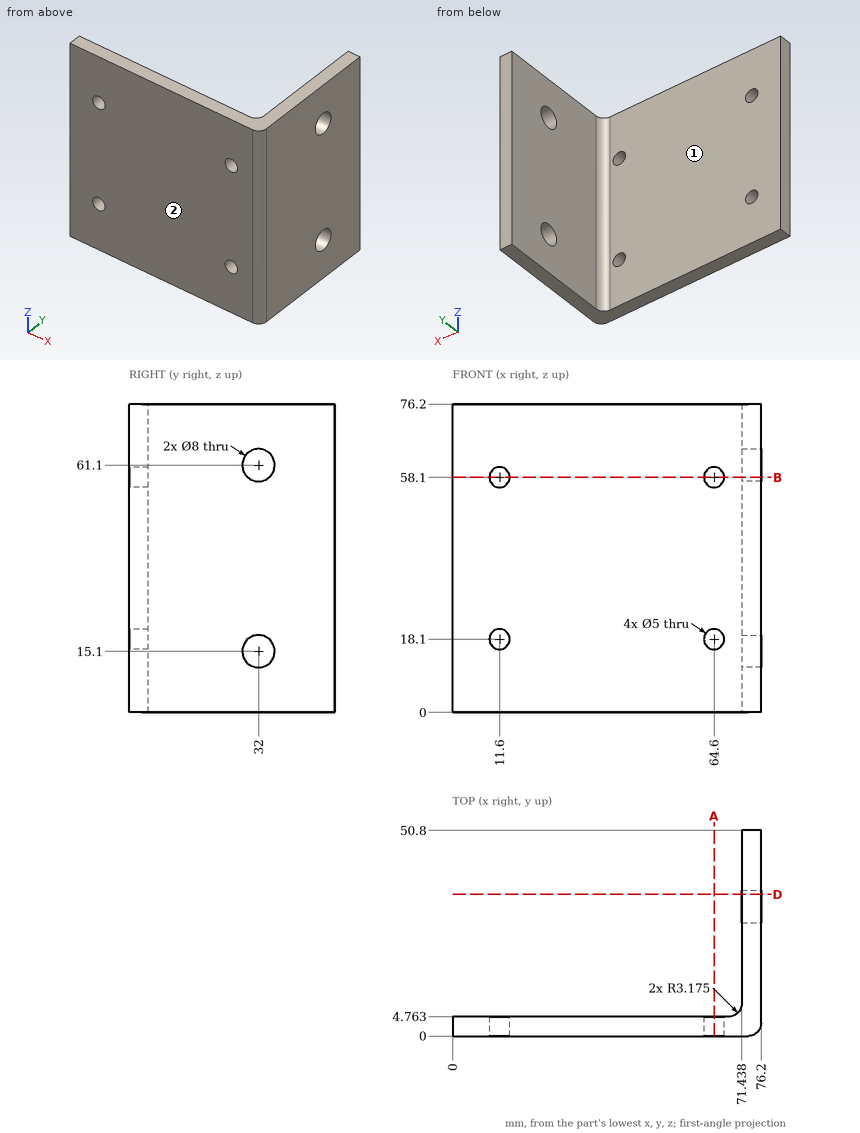
Can you work these out from the drawing? Everything is in mm from the part's minimum corner. A direction names the side the tool comes from. Coordinates: 2 decimals unless noted, no trailing zeros. Loops run counter-clockwise (first coordinate to the right, second up) from the corner with the lowest first, then second, coordinate; pieces in that order, holes last.
1. Imagine slicing it at A-A, the plane x = 64.6. Please give me the cut outline in (y, z).
2. Imagine slicing it at B-B, the plane z = 58.1. Count the separate pieces of the cut face and the enclosed holes in it.
3. Imagine slicing it at D-D, the plane y = 35. Please give me the cut outline in (x, z) (1 decimal).
4. I need wall thicknesses on L1, parallel to Z at x = 64.6, y = 1.85; L2, parallel to X at y = 3, z = 58 (1 decimal); L3, parallel to Z at x = 64, y = 2. Which ranges of each line are inside material? Lowest first, please.
5. For the marked faces 1 and 2, which set-ups out of +Z, -Z, +X, -X, +Y, -Y let a thin tool reach every point of the face, with its end or its side?
6. For P1, Ø1.5, axis at x = 61.5, z = 39, coming from the +Y side; P2, Ø6.5, axis at y = 32, z = 61.1, coming from the +X side; P3, Ø6, axis at x = 64.6, z = 18.1, coming from the -Y side; P4, Ø21.5, axis at y = 20, z = 32.5, coming from the -X side, each with a flat end and sliding along its axis, tell me the tip position at first contact or that it passes through.
Taken from the geometry:
1. outline: (0, 0) - (4.76, 0) - (4.76, 15.6) - (0, 15.6) - close; (0, 20.6) - (4.76, 20.6) - (4.76, 55.6) - (0, 55.6) - close; (0, 60.6) - (4.76, 60.6) - (4.76, 76.2) - (0, 76.2) - close
2. separate pieces: 4
2. enclosed holes: 0
3. outline: (71.4, 0) - (76.2, 0) - (76.2, 12.5) - (71.4, 12.5) - close; (71.4, 17.7) - (76.2, 17.7) - (76.2, 58.5) - (71.4, 58.5) - close; (71.4, 63.7) - (76.2, 63.7) - (76.2, 76.2) - (71.4, 76.2) - close
4. L1: z = 0 to 15.6, 20.6 to 55.6, 60.6 to 76.2
4. L2: x = 0 to 9.1, 14.1 to 62.1, 67.1 to 76.2
4. L3: z = 0 to 15.67, 20.53 to 55.67, 60.53 to 76.2
5. face 1: +Z, -Z, -X, +Y
5. face 2: +Z, -Z, +X, -X, -Y
6. P1: stops at y = 4.76
6. P2: passes through
6. P3: stops at y = 0
6. P4: stops at x = 71.44
